For this review, use the dimensioned drawing (mm, ordinates from the lowest corner) and the shaded views. A direction names the side the tool comes from. Round coordinates to 2 decimals unless told otherwise and drop trailing zeros. Loops run counter-clockwise (first coordinate to the right, second up) from the corner with the lowest first, then second, coordinate; pieces in that order, holes last. Notation, with made-up numbers: (20.25, -37) - (35.25, -37) arc R36 cw to (35.25, 2) - close; hole circle Ø7 at (-25.75, 60.25). An arc over 180 degrees is marked (long way). Return JSON: item names as keys, results as strings. Group by question number.
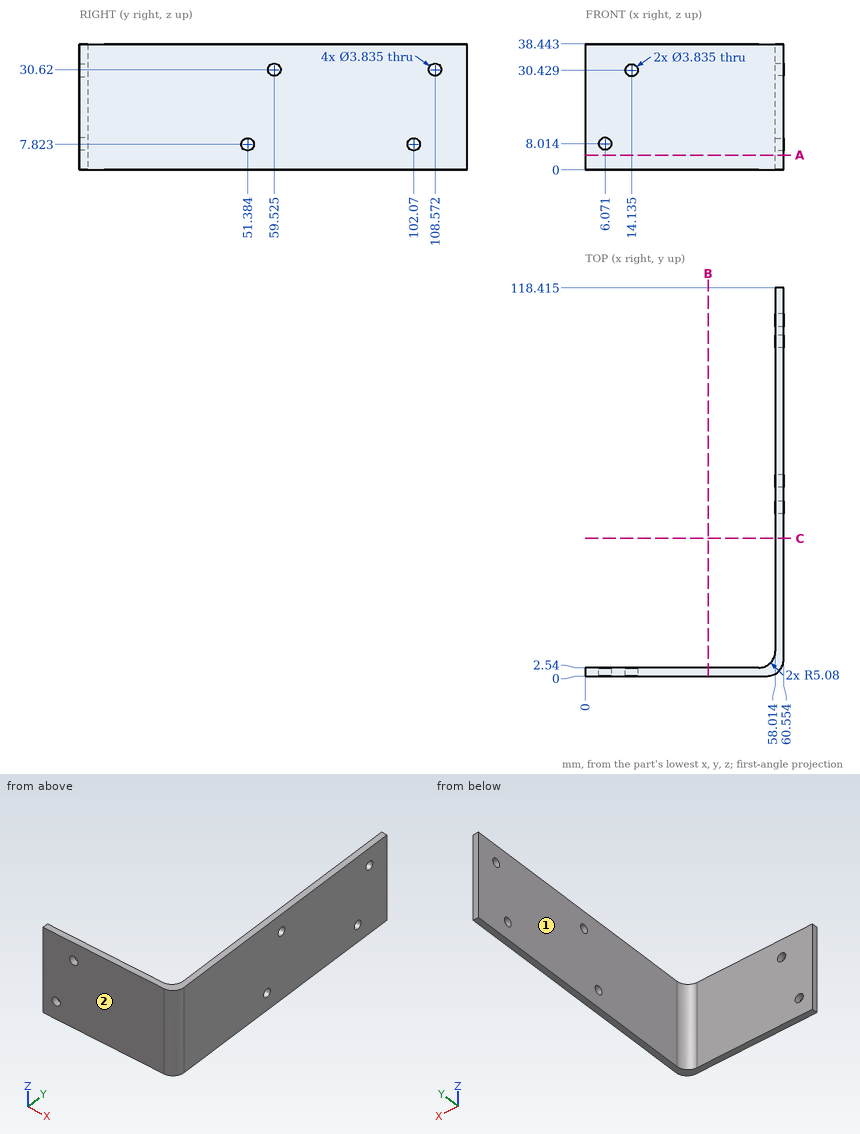
Q1. Add section B-B, the plane x = 37.5. State the section outline as (y, z) points.
Q2. Tool access review of the marked faces 1 and 2: name each direction out of +Z, -Z, +X, -X, +Y, -Y from which nothing blocks a thin tool from reaching the whole face with its end or side.
Q3. Add section A-A, the plane z = 4.5. State the section outline as (x, y) points (1 decimal).
Q4. Add section C-C, the plane y = 42. State the section outline as (x, z) points.
Q5. Insertion check: pin 1 Ø5 at (y, z) = (108.57, 30.62) entering from -X; pin 2 Ø2.5 at (x, z) = (14.14, 30.43) entering from -Y; pin 3 Ø19 at (x, z) = (34, 25) entering from +Y. Each pin has a flat end and moves straight along its axis. Give the tip position at first contact, or say it passes through.
Q6. For line 1 (Y direction, x = 36.5, z = 14); line 2 (X direction, y = 26, z = 34.5), list the stretches that pass through material, from the lowest coordinate up.
Evaluation:
{
 "1": {"outline": "(0, 0) - (2.54, 0) - (2.54, 38.44) - (0, 38.44) - close"},
 "2": {"face 1": "+Z, -Z, -X, +Y", "face 2": "+Z, -Z, +X, -X, -Y"},
 "3": {"outline": "(0, 0) - (55.5, 0) arc R5.1 ccw to (60.6, 5.1) - (60.6, 118.4) - (58, 118.4) - (58, 7.6) arc R5.1 cw to (52.9, 2.5) - (0, 2.5) - close"},
 "4": {"outline": "(58.01, 0) - (60.55, 0) - (60.55, 38.44) - (58.01, 38.44) - close"},
 "5": {"pin 1": "x = 58.01", "pin 2": "through", "pin 3": "y = 2.54"},
 "6": {"line 1": "0 to 2.54", "line 2": "58.01 to 60.55"}
}
